Verification items for this drawing (mm, ordinates from the low corner). Coordinates: 2 decimals unless noted, no trailing zeros. Loops run counter-clockwise (first coordinate to the right, second up) from the corner with the lowest first, then second, coordinate; pieces in that order, holes last. Notation, with made-up numbers: (23.25, 3) - (36.25, 3) arc R17 ccw to (36.25, 13) - close; hole circle Ø10 at (52.25, 88.25). An arc over 180 degrees is marked (long way). Write each question's results on one line, items separated by ' | '. Start each with the question number.
(1) Material ranges on probe 1 along Y at (x, z) = (76.5, 0.35); probe 2 along X at (y, z) = (46.5, 0.8); probe 3 along Y at (x, z) = (59, 1.45), recorded low to high.
(2) Go/stop test with flat-tipped pins: pin 1 Ø1 at (x, z) = (72, 1) entering from -Y; pin 2 Ø6 at (x, y) = (32.5, 76.5) entering from -Z; pin 3 Ø1 at (y, z) = (94, 1) entering from -X; pin 4 Ø0.6 at (x, z) = (71.5, 1) entering from +Y. Record where each tip stops, or that it passes through.
(3) Sectioned sample at B-B (x = 18.5). Enter the section's corners in (y, z), plus the area to 3 significant figures.
(4) Sectioned sample at A-A (y = 47.5). Enter the section's corners in (x, z).
(5) Sectioned sample at C-C (z = 1.1). State how many separate pieces and enclosed holes the cut face has, plus the area to 3 significant figures.
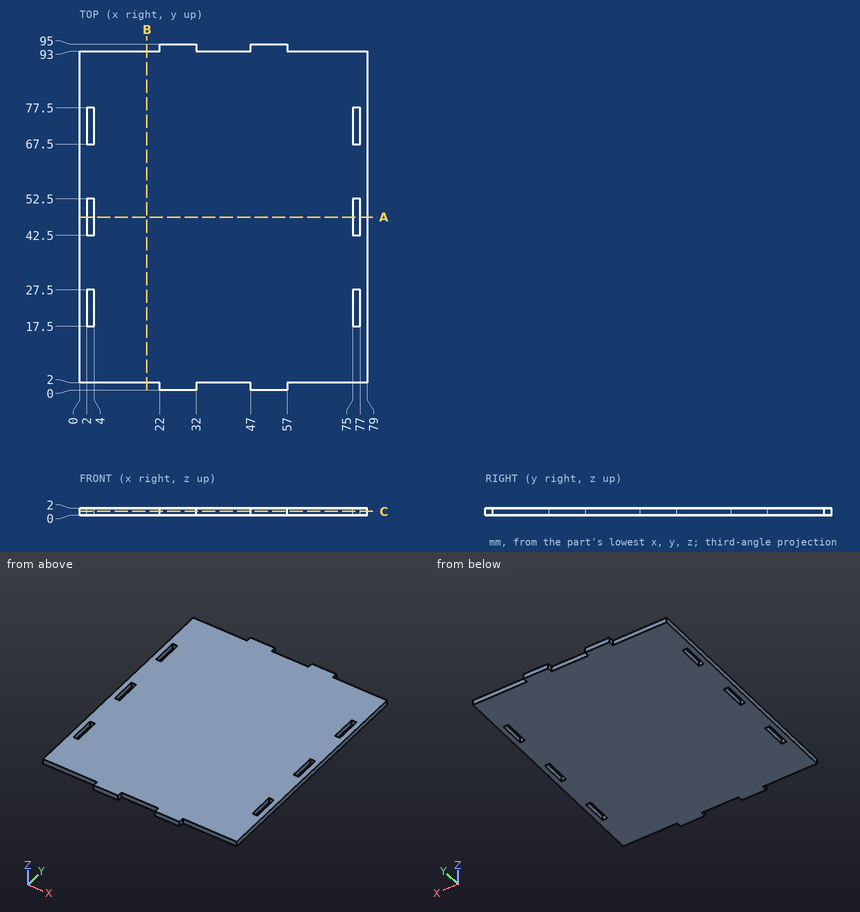
Outcome:
1) probe 1: y = 2 to 17.5, 27.5 to 42.5, 52.5 to 67.5, 77.5 to 93 | probe 2: x = 0 to 2, 4 to 75, 77 to 79 | probe 3: y = 2 to 93
2) pin 1: stops at y = 2 | pin 2: stops at z = 0 | pin 3: stops at x = 22 | pin 4: stops at y = 93
3) outline: (2, 0) - (93, 0) - (93, 2) - (2, 2) - close | area: 182 mm2
4) outline: (0, 0) - (2, 0) - (2, 2) - (0, 2) - close; (4, 0) - (75, 0) - (75, 2) - (4, 2) - close; (77, 0) - (79, 0) - (79, 2) - (77, 2) - close
5) separate pieces: 1 | enclosed holes: 6 | area: 7,150 mm2
